Read the model definition and answer for the solid it produces. Units are mm, in the model's axes. Give positions to 0.01 mm unless a question says otherwise; leave off trailing zeros. Order: outer loops, then holes, each group sorted by start corner. A loop starts at its lowest first (then second) coordinate and runs counter-clockwise, first axis right, second up. Notation, with made-up numbers: (-10, 18.5) - (39, 18.5) arc R6 cw to (39, 23.5) - close; hole circle Ø3 at (78.5, 54.5). An arc over 180 degrees is marked (long way). Use a Markdown table: item, result. Add a question column.
1. Consider L1, parallel to Z at x = -60, y = 7.5; L2, parallel to Z at x = 70, y = 4; L3, parallel to X at y = 6.5, z = -19. Determine where each line is inside the solid, lowest interval first.
2. Flat-ended cylindrical pins translate along their axes: P1, Ø0.8, axis at x = -57, z = -22.5, coming from the -Y side; P2, Ø3, axis at x = -69.5, z = -23.5, coming from the +Y side. Find the tip coordinate at first contact, or state that the pin passes through.
3. A cutting plane is placed at A-A on z = -24. Determine the outline of the cut face in (x, y).
```python
from build123d import *

# Parameters (mm, degrees)
SKETCH1_W           = 175
SKETCH1_H           = 90
BOSS_EXTRUDE1_DEPTH = 10
SKETCH2_W           = 19
SKETCH2_H           = 10.1
CUT_EXTRUDE1_DEPTH  = 5.4
CUT_EXTRUDE2_DEPTH  = 10.1
FILLET1_R           = 1
SKETCH2_8_R         = 1.5
CUT_EXTRUDE3_DEPTH  = 11


with BuildPart() as part:
    # Sketch1 → Boss-Extrude1 (new body)
    with BuildSketch(Plane(origin=(0, 0, 0), x_dir=(1, 0, 0), z_dir=(0, 1, 0))):
        Rectangle(SKETCH1_W, SKETCH1_H)
    extrude(amount=BOSS_EXTRUDE1_DEPTH)

    # Sketch2 → Cut-Extrude1 (cut)
    with BuildSketch(Plane(origin=(0, 10, 0), x_dir=(1, 0, 0), z_dir=(0, 1, 0))):
        with Locations((-67.5, -23.5)):
            Rectangle(SKETCH2_W, SKETCH2_H)
    cut_extrude1 = extrude(amount=-CUT_EXTRUDE1_DEPTH, mode=Mode.SUBTRACT)

    # Sketch7 → Cut-Extrude2 (cut)
    with BuildSketch(Plane.XY.offset(18.45)):
        Polygon((-77, 5), (-77, 10), (-77.662881067, 10), (-77.400415076, 7), (-78.400415076, 7), align=None)
        Polygon((-58, 5), (-58, 10), (-57.337118933, 10), (-57.599584924, 7), (-56.599584924, 7), align=None)
    cut_extrude2 = extrude(amount=CUT_EXTRUDE2_DEPTH, mode=Mode.SUBTRACT)

    # Mirror1: Cut-Extrude1, Cut-Extrude2 across plane
    add(cut_extrude1.mirror(Plane.XY), mode=Mode.SUBTRACT)
    add(cut_extrude2.mirror(Plane.XY), mode=Mode.SUBTRACT)

    # Fillet1
    fillet1_edges = [part.edges().sort_by_distance(p)[0] for p in [
        (-87.5, 5, -45),
        (87.5, 5, -45),
        (87.5, 5, 45),
        (-87.5, 5, 45),
    ]]
    fillet(fillet1_edges, radius=FILLET1_R)

    # Sketch2<8> → Cut-Extrude3 (cut, through all)
    with BuildSketch(Plane(origin=(0, 10, 0), x_dir=(1, 0, 0), z_dir=(0, 1, 0))):
        with Locations((-5, 19)):
            Circle(SKETCH2_8_R)
        with Locations((70, 19)):
            Circle(SKETCH2_8_R)
    extrude(amount=-CUT_EXTRUDE3_DEPTH, mode=Mode.SUBTRACT)


solid = part.part
```
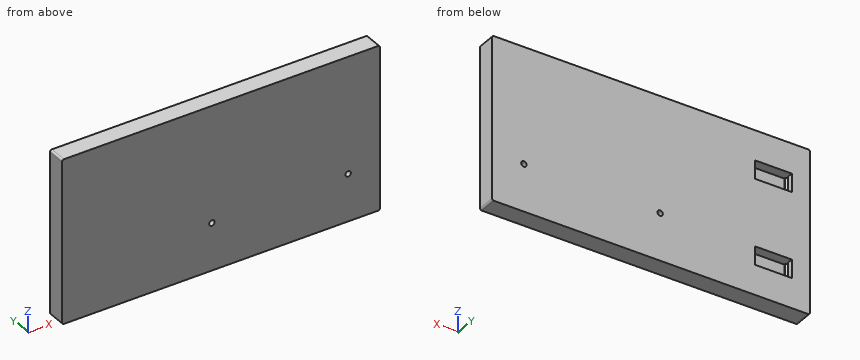
Output values:
| question | item | result |
|---|---|---|
| 1 | L1 | -45 to -28.55, -18.45 to 18.45, 28.55 to 45 |
| 1 | L2 | -45 to -20.5, -17.5 to 45 |
| 1 | L3 | -87.5 to -78.05, -56.95 to -6.5, -3.5 to 68.5, 71.5 to 87.5 |
| 2 | P1 | y = 0 |
| 2 | P2 | y = 4.6 |
| 3 | outline | (-87.5, 0) - (87.5, 0) - (87.5, 10) - (-57.34, 10) - (-57.6, 7) - (-56.6, 7) - (-58, 5) - (-58, 4.6) - (-77, 4.6) - (-77, 5) - (-78.4, 7) - (-77.4, 7) - (-77.66, 10) - (-87.5, 10) - close |
